```python
from build123d import *

# Parameters (mm, degrees)
F0_W      = 101.6
F0_H      = 50.8
F1_DEPTH  = 19.05
F2_R      = 2.54
F4_D      = 2.5
F4_DEPTH  = 14.2
F4_TIP    = 0.7510757738
F6_DEPTH  = 5.715
F8_D      = 2.5
F8_DEPTH  = 11.66
F8_TIP    = 0.7510757738
F10_DEPTH = 9.525
F12_D     = 2.5
F12_DEPTH = 3.81
F12_TIP   = 0.7510757738


with BuildPart() as f1:
    # F0 (on Top) → F1 (new body)
    with BuildSketch(Plane.XY):
        Rectangle(F0_W, F0_H)
    extrude(amount=-F1_DEPTH)

    # F2
    f2_edges = [f1.edges().sort_by_distance(p)[0] for p in [
        (-50.8, -25.4, -9.525),
        (50.8, -25.4, -9.525),
        (50.8, 25.4, -9.525),
        (-50.8, 25.4, -9.525),
    ]]
    fillet(f2_edges, radius=F2_R)

    # F4
    with Locations(Plane.XY):
        with Locations((-46.355, 20.955), (46.355, 20.955), (46.355, -20.955), (-46.355, -20.955)):
            Hole(F4_D / 2, depth=F4_DEPTH)
            with Locations((0, 0, -(F4_DEPTH + F4_TIP / 2))):  # 118° drill point
                Cone(0, F4_D / 2, F4_TIP, mode=Mode.SUBTRACT)

    # F5 (on face) → F6 (cut)
    with BuildSketch(Plane.XY):
        with BuildLine():
            Line((-40.005, -23.8125), (40.005, -23.8125))
            ThreePointArc((40.005, -23.8125), (42.2500640303, -22.8825640303), (43.18, -20.6375))
            Line((43.18, -20.6375), (43.18, 20.6375))
            ThreePointArc((43.18, 20.6375), (42.2500640303, 22.8825640303), (40.005, 23.8125))
            Line((40.005, 23.8125), (-40.005, 23.8125))
            ThreePointArc((-40.005, 23.8125), (-42.2500640303, 22.8825640303), (-43.18, 20.6375))
            Line((-43.18, 20.6375), (-43.18, -20.6375))
            ThreePointArc((-43.18, -20.6375), (-42.2500640303, -22.8825640303), (-40.005, -23.8125))
        make_face()
    extrude(amount=-F6_DEPTH, mode=Mode.SUBTRACT)

    # F8
    with Locations(Plane.XY.offset(-5.715)):
        with Locations((-38.4048, 20.6248), (27.8892, 20.6248), (27.8892, -20.6248), (-38.4048, -20.6248)):
            Hole(F8_D / 2, depth=F8_DEPTH)
            with Locations((0, 0, -(F8_DEPTH + F8_TIP / 2))):  # 118° drill point
                Cone(0, F8_D / 2, F8_TIP, mode=Mode.SUBTRACT)

    # F9 (on face) → F10 (cut)
    with BuildSketch(Plane.XY.offset(-5.715)):
        with BuildLine():
            Line((34.2391873, -23.8125), (40.005, -23.8125))
            ThreePointArc((40.005, -23.8125), (42.2500640303, -22.8825640303), (43.18, -20.6375))
            Line((43.18, -20.6375), (43.18, 20.6375))
            ThreePointArc((43.18, 20.6375), (42.2500640303, 22.8825640303), (40.005, 23.8125))
            Line((40.005, 23.8125), (34.2391873, 23.8125))
            ThreePointArc((34.2391873, 23.8125), (31.9918793271, 22.8803178426), (31.06419365, 20.63115))
            ThreePointArc((31.06419365, 20.63115), (27.8892, 17.4498), (24.71420635, 20.63115))
            ThreePointArc((24.71420635, 20.63115), (23.7865206729, 22.8803178426), (21.5392127, 23.8125))
            Line((21.5392127, 23.8125), (-32.0548127, 23.8125))
            ThreePointArc((-32.0548127, 23.8125), (-34.3021206729, 22.8803178426), (-35.22980635, 20.63115))
            ThreePointArc((-35.22980635, 20.63115), (-36.4606005283, 18.1146778089), (-39.2049, 17.5522660311))
            ThreePointArc((-39.2049, 17.5522660311), (-41.9466883761, 16.9917971987), (-43.18, 14.4797320622))
            Line((-43.18, 14.4797320622), (-43.18, -14.4797320622))
            ThreePointArc((-43.18, -14.4797320622), (-41.9466883761, -16.9917971987), (-39.2049, -17.5522660311))
            ThreePointArc((-39.2049, -17.5522660311), (-36.4606005283, -18.1146778089), (-35.22980635, -20.63115))
            ThreePointArc((-35.22980635, -20.63115), (-34.3021206729, -22.8803178426), (-32.0548127, -23.8125))
            Line((-32.0548127, -23.8125), (21.5392127, -23.8125))
            ThreePointArc((21.5392127, -23.8125), (23.7865206729, -22.8803178426), (24.71420635, -20.63115))
            ThreePointArc((24.71420635, -20.63115), (27.8892, -17.4498), (31.06419365, -20.63115))
            ThreePointArc((31.06419365, -20.63115), (31.9918793271, -22.8803178426), (34.2391873, -23.8125))
        make_face()
    extrude(amount=-F10_DEPTH, mode=Mode.SUBTRACT)

    # F12
    with Locations(Plane.XY.offset(-15.24)):
        with Locations((-16.9418, 18.7325), (-16.9418, 13.6525), (-16.9418, 8.5725), (-16.9418, 3.4925), (-16.9418, -1.5875), (-16.9418, -6.6675), (6.4262, -6.6675), (6.4262, -1.5875), (6.4262, 3.4925), (6.4262, 8.5725), (6.4262, 13.6525), (6.4262, 18.7325)):
            Hole(F12_D / 2, depth=F12_DEPTH)
            with Locations((0, 0, -(F12_DEPTH + F12_TIP / 2))):  # 118° drill point
                Cone(0, F12_D / 2, F12_TIP, mode=Mode.SUBTRACT)


solid = f1.part
```
Here's how the part is built. I have some questions about the finished solid (model axes, mm). A direction names the side the tool comes from. Coordinates: 2 decimals unless noted, no trailing zeros. Loops run counter-clockwise (first coordinate to the right, second up) from the corner with the lowest first, then second, coordinate; pieces in that order, holes last. Notation, with made-up numbers: (71, -11.5) - (88, -11.5) arc R17 cw to (88, -7.5) - close; hole circle Ø10 at (-10, 15.25). An arc over 180 degrees is marked (long way). Return JSON: item names as keys, results as strings. Group by question number.
Item 1: On a 3-axis mill with a long thin cutter (end or side, diameter ignored), from which of +Z, -Z, +X, -X, +Y, -Y can I reach the whole of each face in a straight line? I mean faces 4 (the face through (6.59, 19.97, -17.17)), 5 (the face through (-42.225, 22.907, -2.817)). Say none if no direction works.
Item 2: Will these pins go through, and if not, where does the flat tip stop? P1, Ø2, axis at x = -46.355, y = -20.955, coming from the +Z side; P2, Ø1, axis at x = -35.5, y = -3, coming from the +Z side; P3, Ø1.5, axis at x = -46.355, y = 20.955, coming from the +Z side.
Item 3: I need wall thicknesses on line 1 (Y direction, x = 16, z = -0.75); line 2 (X direction, y = 9.5, z = -11.25); line 3 (Y direction, x = -38, z = -16.5). Which ranges of each line are inside material? Lowest first, please. Write a range as from..to.
Item 4: If we section it at A-A on x = 18: Write out the boundary of the cut face in (y, z), and give its area (3 significant figures).
Item 5: We'd pull the mould along X, two halves only. Please class faces 1 (the face through (-50.076, -24.636, -9.658)), 2 (the face through (42.27, 22.86, -7.51)), 3 (the face through (0, -24, 0)): +X half, -X half, draft (parallel to the pull), parting line (faces both ways), or undercut.
Item 6: If we section it at B-B on z = -1.25: State how many separate pieces and enclosed holes the cut face has, and give its area (3 significant figures).
Item 7: If we section it at C-C on x = 42: Write out the boundary of the cut face in (y, z), and give its area (3 significant figures).
Calculated:
{
 "1": {"face 4": "+Z, -Z", "face 5": "+Z"},
 "2": {"P1": "stops at z = -14.35", "P2": "stops at z = -15.24", "P3": "stops at z = -14.5"},
 "3": {"line 1": "y = -25.4..-23.81, 23.81..25.4", "line 2": "x = -50.8..-43.18, 43.18..50.8", "line 3": "y = -25.4..-21.81, -19.44..19.44, 21.81..25.4"},
 "4": {"outline": "(-25.4, -19.05) - (25.4, -19.05) - (25.4, 0) - (23.81, 0) - (23.81, -15.24) - (-23.81, -15.24) - (-23.81, 0) - (-25.4, 0) - close", "area": "242 mm^2"},
 "5": {"face 1": "-X half", "face 2": "undercut", "face 3": "draft"},
 "6": {"separate pieces": "1", "enclosed holes": "5", "area": "1,030 mm^2"},
 "7": {"outline": "(-25.4, -19.05) - (25.4, -19.05) - (25.4, 0) - (23.11, 0) - (23.11, -15.24) - (-23.11, -15.24) - (-23.11, 0) - (-25.4, 0) - close", "area": "263 mm^2"}
}
